Design review of the part built by this model. Coordinates are the model's own, in mm. Face numbers are marked on the shaded views. A direction names the side the tool comes from. Coordinates: 2 decimals unless noted, no trailing zeros. Loops run counter-clockwise (first coordinate to the right, second up) from the corner with the lowest first, then second, coordinate; pieces in that order, holes last. Notation, with made-up numbers: (72.5, -5.5) -> (109.5, -5.5) arc R28 ccw to (109.5, 17.5) -> close; hole circle Ø9 at (8.5, 81). An arc over 180 degrees is marked (long way). One line per item, written item: value. Start each with the question number.
1. Add section D-D on x = -21.5. Write out the cut boundary in (y, z).
2. Machinability: for the marked faces 4 and 5, which of the approach directions +Z, -Z, +X, -X, +Y, -Y give a long, thin tool a straight path to every point of the face, cutting with its end or side? Answer none if there is none.
3. For probe 1 along Y at (x, z) = (-15.25, 14); probe 2 along X at (y, z) = (6.5, 12.5); probe 3 along X at (y, z) = (12.5, -0.5), list the stretches that pass through material, from the lowest coordinate up.
4. Add section A-A on z = 13.25. Write out the cut boundary in (x, y).
5. Add section C-C on x = -11.25. Write out the cut boundary in (y, z).
6. Add section B-B on y = 13.75. Write out the cut boundary in (x, z), plus the area to 3 significant figures.
7. Draft analysis for pull direction X (two halves, no side actions). For the marked faces 1, 2 and 3, state which applies: pulls with the +X half, pulls with the -X half, needs draft (parallel to the pull), parting line crosses it, or undercut.
```python
from build123d import *

# Parameters (mm, degrees)
F0_W        = 23.3
F0_H        = 22.7
F1_DEPTH    = 15
F2_T        = 2
F3_T1_DEPTH = 32
F5_DEPTH    = 25


# Not quite as in the source:
# - a fillet or chamfer that OpenCascade refuses, or shapes differently, is made with other operations: its cross-section is extruded or revolved along the edge and cut away or added


with BuildPart() as f1:
    # F0 (on Top) → F1 (new body)
    with BuildSketch(Plane.XY):
        with Locations((-11.65, 11.35)):
            Rectangle(F0_W, F0_H)
    extrude(amount=F1_DEPTH)

    # F2
    f2_openings = [f1.faces().sort_by_distance(p)[0] for p in [
        (-11.65, 11.35, 15),
    ]]
    offset(amount=F2_T, openings=f2_openings, kind=Kind.INTERSECTION)

    # F3: fillet of radius 3 on 4 edges, made by hand

    # F3_s2 → F3_t1 (cut)
    with BuildSketch(Plane.XY.offset(-9.5)):
        with BuildLine():
            ThreePointArc((-22.3, -2), (-24.4213203436, -1.1213203436), (-25.3, 1))
            Line((-25.3, 1), (-25.3, -2))
            Line((-25.3, -2), (-22.3, -2))
        make_face()
        with BuildLine():
            ThreePointArc((-1, -2), (1.1213203436, -1.1213203436), (2, 1))
            Line((2, 1), (2, -2))
            Line((2, -2), (-1, -2))
        make_face()
        with BuildLine():
            ThreePointArc((2, 21.7), (1.1213203436, 23.8213203436), (-1, 24.7))
            Line((-1, 24.7), (2, 24.7))
            Line((2, 24.7), (2, 21.7))
        make_face()
        with BuildLine():
            ThreePointArc((-22.3, 24.7), (-24.4213203436, 23.8213203436), (-25.3, 21.7))
            Line((-25.3, 21.7), (-25.3, 24.7))
            Line((-25.3, 24.7), (-22.3, 24.7))
        make_face()
    extrude(amount=F3_T1_DEPTH, mode=Mode.SUBTRACT)

    # F4 (on face) → F5 (cut)
    with BuildSketch(Plane(origin=(0, 0, -2), x_dir=(1, 0, 0), z_dir=(0, 0, -1))):
        Polygon((-18.8904213403, -15.5302592099), (-11.65, -19.7105184197), (-4.4095786597, -15.5302592099), (-4.4095786597, -7.1697407901), (-11.65, -2.9894815803), (-18.8904213403, -7.1697407901), align=None)
    extrude(amount=-F5_DEPTH, mode=Mode.SUBTRACT)


solid = f1.part
```
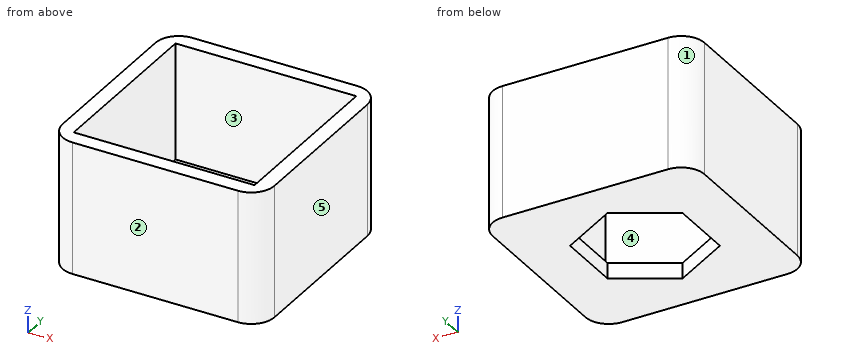
Worked answers:
1. outline: (-2, -2) -> (24.7, -2) -> (24.7, 15) -> (22.7, 15) -> (22.7, 0) -> (0, 0) -> (0, 15) -> (-2, 15) -> close
2. face 4: +Z
2. face 5: +Z, -Z, +X, +Y, -Y
3. probe 1: y = -2 to 0, 22.7 to 24.7
3. probe 2: x = -25.3 to -23.3, 0 to 2
3. probe 3: x = -25.3 to -18.89, -4.41 to 2
4. outline: (-25.3, 1) arc R3 ccw to (-22.3, -2) -> (-1, -2) arc R3 ccw to (2, 1) -> (2, 21.7) arc R3 ccw to (-1, 24.7) -> (-22.3, 24.7) arc R3 ccw to (-25.3, 21.7) -> close; hole (-23.3, 0) -> (0, 0) -> (0, 22.7) -> (-23.3, 22.7) -> close
5. outline: (-2, -2) -> (3.22, -2) -> (3.22, 0) -> (0, 0) -> (0, 15) -> (-2, 15) -> close; (19.48, -2) -> (24.7, -2) -> (24.7, 15) -> (22.7, 15) -> (22.7, 0) -> (19.48, 0) -> close
6. outline: (-25.3, -2) -> (-18.89, -2) -> (-18.89, 0) -> (-23.3, 0) -> (-23.3, 15) -> (-25.3, 15) -> close; (-4.41, -2) -> (2, -2) -> (2, 15) -> (0, 15) -> (0, 0) -> (-4.41, 0) -> close
6. area: 85.6 mm²
7. face 1: pulls with the -X half
7. face 2: needs draft
7. face 3: undercut
